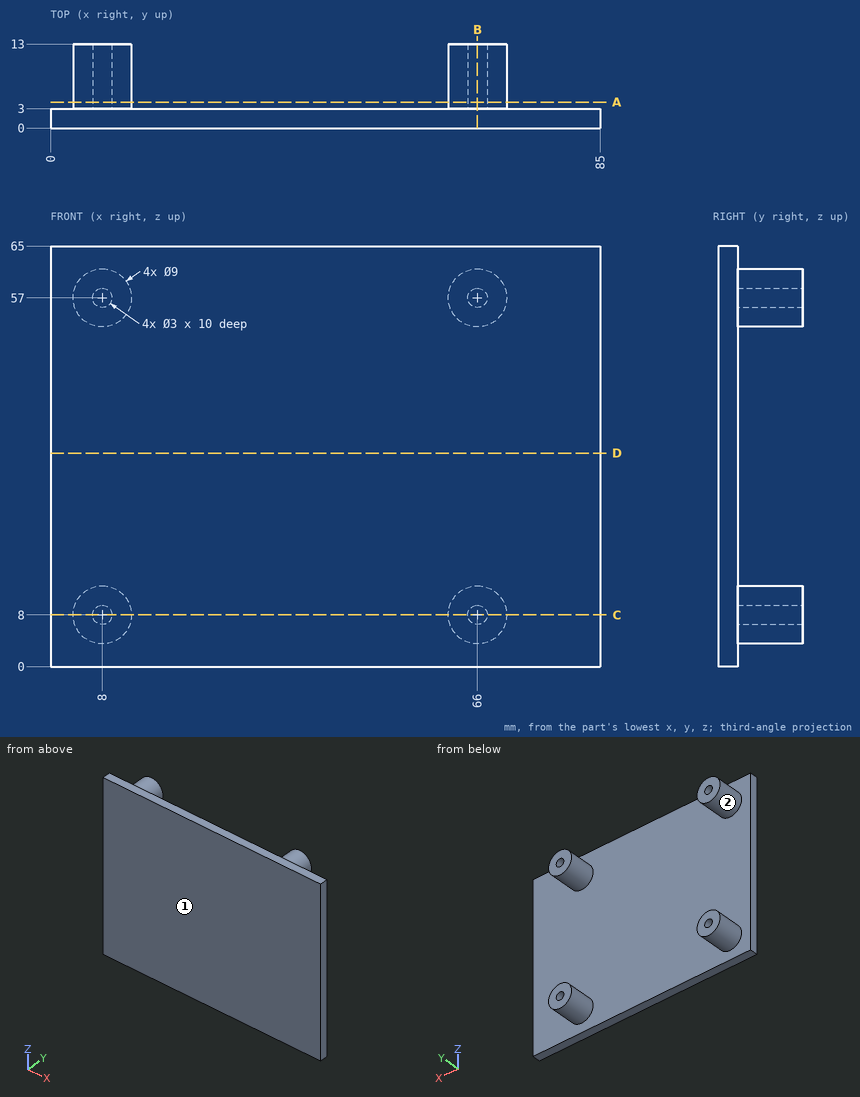
Study the drawing (mm; zero at the part's minimum x, y, z) and answer. Give positions to 0.01 mm unless a question says otherwise; leave off trailing zeros. Write each loop counter-clockwise with the first axis right and the second up, starting at its lowest first coordinate (ties: lowest second). Pieces come first, ordered by that corner, then holes.
Item 1: Determine the mould class of the marked faces 1 and 2 for opening direction X: released by +X, released by -X, zero draft, split by the parting line, or undercut.
Item 2: Section C-C, the plane z = 8 is taken. Write down the section's boundary in (x, y).
Item 3: A flat-ended cylindrical pin translates along its axis: P1, Ø2.5, axis at x = 66, z = 57, coming from the +Y side. Find the tip coordinate at first contact, or state that the pin passes through.
Item 4: Section D-D, the plane z = 33 is taken. Write down the section's boundary in (x, y), plus the area to 3 significant figures.
Item 5: Find the intervals of material crossed by line 1 along X through (y, z) = (7, 57); line 2 along X through (y, z) = (10.75, 57.5); line 3 along Y through (x, z) = (66, 18.5), in increasing order.
Item 6: Section B-B, the plane x = 66 is taken. Write down the section's boundary in (y, z).
Item 7: Section A-A, the plane y = 4 is taken. Write down the section's boundary in (x, z), plus the area to 3 significant figures.
Completed:
1. face 1: zero draft
1. face 2: undercut
2. outline: (0, 0) - (85, 0) - (85, 3) - (70.5, 3) - (70.5, 13) - (67.5, 13) - (67.5, 3) - (64.5, 3) - (64.5, 13) - (61.5, 13) - (61.5, 3) - (12.5, 3) - (12.5, 13) - (9.5, 13) - (9.5, 3) - (6.5, 3) - (6.5, 13) - (3.5, 13) - (3.5, 3) - (0, 3) - close
3. P1: stops at y = 3
4. outline: (0, 0) - (85, 0) - (85, 3) - (0, 3) - close
4. area: 255 mm2
5. line 1: x = 3.5 to 6.5, 9.5 to 12.5, 61.5 to 64.5, 67.5 to 70.5
5. line 2: x = 3.53 to 6.59, 9.41 to 12.47, 61.53 to 64.59, 67.41 to 70.47
5. line 3: y = 0 to 3
6. outline: (0, 0) - (3, 0) - (3, 3.5) - (13, 3.5) - (13, 6.5) - (3, 6.5) - (3, 9.5) - (13, 9.5) - (13, 12.5) - (3, 12.5) - (3, 52.5) - (13, 52.5) - (13, 55.5) - (3, 55.5) - (3, 58.5) - (13, 58.5) - (13, 61.5) - (3, 61.5) - (3, 65) - (0, 65) - close
7. outline: circle Ø9 at (8, 8); circle Ø9 at (8, 57); circle Ø9 at (66, 8); circle Ø9 at (66, 57); hole circle Ø3 at (8, 8); hole circle Ø3 at (8, 57); hole circle Ø3 at (66, 8); hole circle Ø3 at (66, 57)
7. area: 226 mm2
